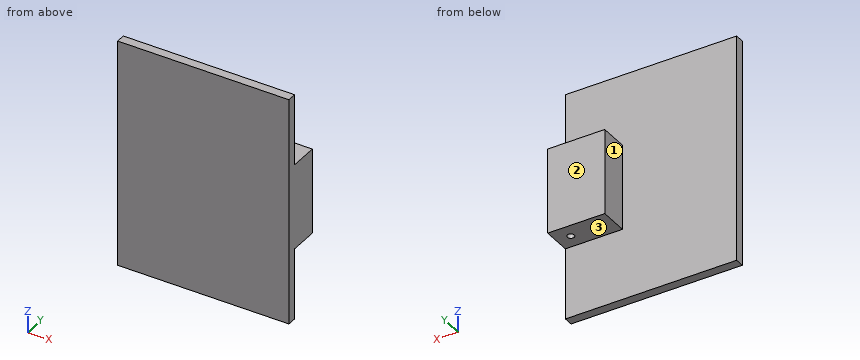
from build123d import *

# Parameters (mm, degrees)
SKETCH1_W               = 300
SKETCH1_H               = 400
BOSS_EXTRUDE1_DEPTH     = 16
SKETCH2_W               = 100
SKETCH2_H               = 150
BOSS_EXTRUDE2_DEPTH     = 50
CUT_EXTRUDE1_DEPTH      = 321.126537482
CUT_EXTRUDE1_DEPTH_BACK = 321.126537482
SKETCH3_R               = 6


with BuildPart() as part:
    # Sketch1 → Boss-Extrude1 (new body)
    with BuildSketch(Plane(origin=(0, 0, 0), x_dir=(1, 0, 0), z_dir=(0, 1, 0))):
        Rectangle(SKETCH1_W, SKETCH1_H)
    extrude(amount=BOSS_EXTRUDE1_DEPTH)

    # Sketch2 → Boss-Extrude2 (add)
    with BuildSketch(Plane(origin=(0, 16, 0), x_dir=(1, 0, 0), z_dir=(0, 1, 0))):
        with Locations((100, 0)):
            Rectangle(SKETCH2_W, SKETCH2_H)
    extrude(amount=BOSS_EXTRUDE2_DEPTH)

    # Sketch3 → Cut-Extrude1 (cut, two sides: drawn at the far end of the back side and taken through both)
    with BuildSketch(Plane(origin=(0, 0, -75), x_dir=(-1, 0, 0), z_dir=(0, 0, -1)).offset(-CUT_EXTRUDE1_DEPTH_BACK)):
        with Locations((-125, 41)):
            Circle(SKETCH3_R)
    extrude(amount=CUT_EXTRUDE1_DEPTH + CUT_EXTRUDE1_DEPTH_BACK, mode=Mode.SUBTRACT)


solid = part.part
Work out the finished part from the listing and answer in its coordinate system (mm). Face numbers are marked on the shaded views. A direction names the side the tool comes from. Coordinates: 2 decimals unless noted, no trailing zeros. Loops run counter-clockwise (first coordinate to the right, second up) from the corner with the lowest first, then second, coordinate; pieces in that order, holes last. Notation, with made-up numbers: M 54,9 L 71,9 A30 ccw 71,31 Z; hole C -26.5,19.5 d3. An arc over 180 degrees is marked long. Answer in a Markdown table with one row per item. Add a question column.
1. A tool of negligible diameter and unlimited length cuts with its end or side. For the marked faces 1, 2 and 3, from which of +Z, -Z, +X, -X, +Y, -Y can it reach the whole face along a straight path? Write none if from no direction.
2. Find section B-B, the plane y = 41. Write down the section's boundary in (x, z), then the cut area to 3 significant figures.
3. Find section D-D, the plane x = 65.5. Write down the section's boundary in (y, z), then the cut area to 3 significant figures.
4. Find section C-C, the plane z = -47. Write down the section's boundary in (x, y).
5. Consider L1, parallel to X at y = 41, z = 35; L2, parallel to Y at x = 125, z = 29; L3, parallel to Z at x = 93, y = 20. Determine where each line is inside the solid, lowest interval first.
6. Find section A-A, the plane x = 125. Write down the section's boundary in (y, z), then the cut area to 3 significant figures.
7. Flat-ended cylindrical pins translate along their axes: P1, Ø10, axis at x = 95, z = -109, coming from the +Y side; P2, Ø2, axis at x = -81, z = 131, coming from the -Y side; P3, Ø25, axis at y = 46, z = 26, coming from the -X side; P4, Ø15, axis at x = 105.5, y = 37, coming from the -Z side. Find the tip coordinate at first contact, or state that the pin passes through.
Reported:
| question | item | result |
|---|---|---|
| 1 | face 1 | +Z, -Z, -X, +Y |
| 1 | face 2 | +Z, -Z, +X, -X, +Y |
| 1 | face 3 | -Z, +X, -X, +Y |
| 2 | outline | M 50,-75 L 119,-75 L 119,75 L 50,75 Z; M 131,-75 L 150,-75 L 150,75 L 131,75 Z |
| 2 | area | 13,200 mm^2 |
| 3 | outline | M 0,-200 L 16,-200 L 16,-75 L 66,-75 L 66,75 L 16,75 L 16,200 L 0,200 Z |
| 3 | area | 13,900 mm^2 |
| 4 | outline | M -150,0 L 150,0 L 150,66 L 50,66 L 50,16 L -150,16 Z; hole C 125,41 d12 |
| 5 | L1 | x = 50 to 119, 131 to 150 |
| 5 | L2 | y = 0 to 35, 47 to 66 |
| 5 | L3 | z = -75 to 75 |
| 6 | outline | M 0,-200 L 16,-200 L 16,-75 L 35,-75 L 35,75 L 16,75 L 16,200 L 0,200 Z; M 47,-75 L 66,-75 L 66,75 L 47,75 Z |
| 6 | area | 12,100 mm^2 |
| 7 | P1 | stops at y = 16 |
| 7 | P2 | stops at y = 0 |
| 7 | P3 | stops at x = 50 |
| 7 | P4 | stops at z = -75 |
